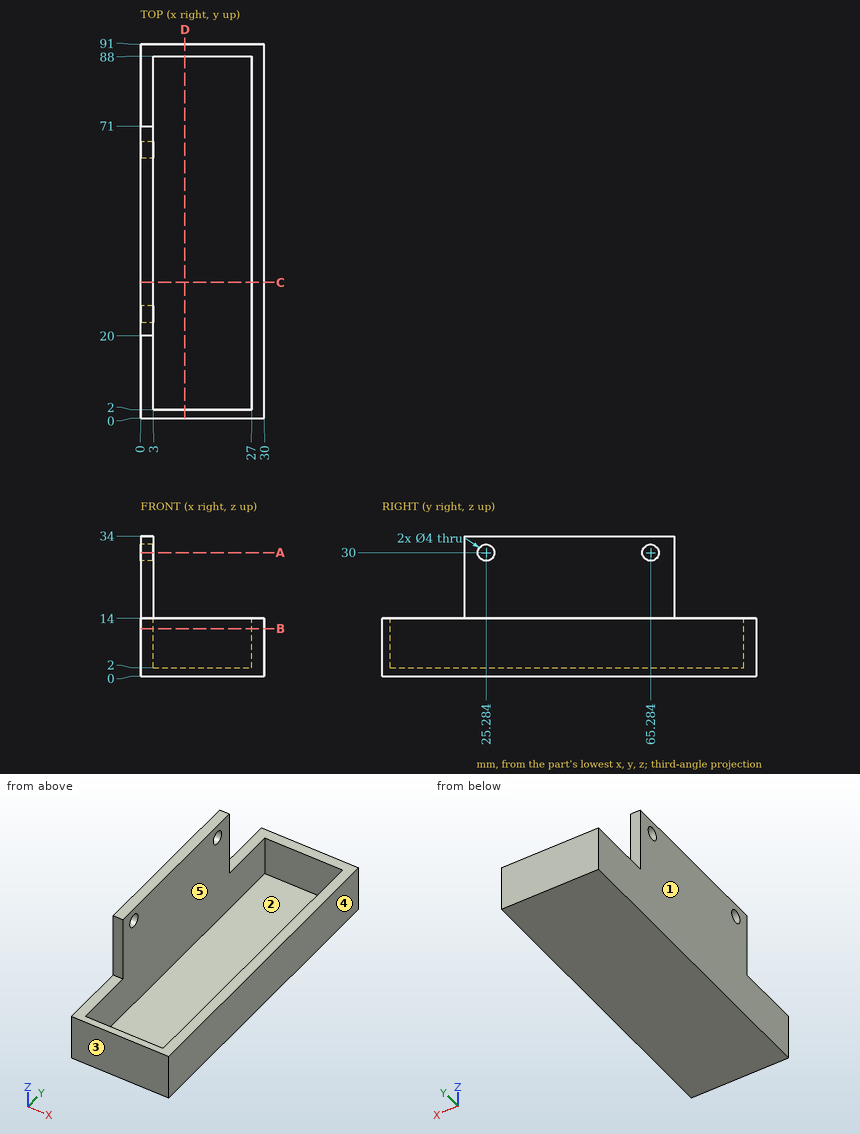
Here's the drawing with two shaded views (mm, measured from the low corner). I have some questions. A direction names the side the tool comes from. Coordinates: 2 decimals unless noted, no trailing zeros. Order: outer loops, then holes, each group sorted by start corner. A loop starts at its lowest first (then second) coordinate and runs counter-clockwise, first axis right, second up.
Q1. Thinking about a two-plate mould opening in Y: for the marked faces 1, 2 and 3, which applies, released by +Y, released by -Y, zero draft, split by the parting line, or undercut?
Q2. Please list where these lines run through material, in increasing order: L1, parallel to X at y = 68, z = 3.5; L2, parallel to Y at x = 15.25, z = 7; L3, parallel to X at y = 44, z = 29.5.
Q3. Suppose I cut it at D-D on x = 10.75. Please give me the cut outline in (y, z).
Q4. Which directions (+Z, -Z, +X, -X, +Y, -Y) give clear straight access to the entire face, cutting with the end or side of a thin tool? Please do the marked faces 4 and 5.
Q5. Suppose I cut it at C-C on y = 33. Please give me the cut outline in (x, z), and give its area (3 significant figures).
Q6. Suppose I cut it at A-A on z = 30. Please give me the cut outline in (x, y) (1 decimal), and give its area (3 significant figures).
Q7. Will these pins go through, and if not, where does the flat tip stop? pin 1 (5 mm diameter, centred on y = 25.28, z = 30, fed in from +X); pin 2 (2.5 mm diameter, centred on x = 2, z = 26, fed in from +Y); pin 3 (12 mm diameter, centred on x = 11, y = 38.5, fed in from +Z).
Q8. Suppose I cut it at B-B on z = 11.5. Please give me the cut outline in (x, y), and give its area (3 significant figures).
Answer:
1. face 1: zero draft
1. face 2: undercut
1. face 3: released by -Y
2. L1: x = 0 to 3, 27 to 30
2. L2: y = 0 to 2, 88 to 91
2. L3: x = 0 to 3
3. outline: (0, 0) - (91, 0) - (91, 14) - (88, 14) - (88, 2) - (2, 2) - (2, 14) - (0, 14) - close
4. face 4: +Z, -Z, +X, +Y, -Y
4. face 5: +Z
5. outline: (0, 0) - (30, 0) - (30, 14) - (27, 14) - (27, 2) - (3, 2) - (3, 34) - (0, 34) - close
5. area: 192 mm2
6. outline: (0, 20) - (3, 20) - (3, 23.3) - (0, 23.3) - close; (0, 27.3) - (3, 27.3) - (3, 63.3) - (0, 63.3) - close; (0, 67.3) - (3, 67.3) - (3, 71) - (0, 71) - close
6. area: 129 mm2
7. pin 1: stops at x = 3
7. pin 2: stops at y = 71
7. pin 3: stops at z = 2
8. outline: (0, 0) - (30, 0) - (30, 91) - (0, 91) - close; hole (3, 2) - (27, 2) - (27, 88) - (3, 88) - close
8. area: 666 mm2
